```python
from build123d import *

# Parameters (mm, degrees)
CUT_EXTRUDE1_DEPTH = 2.5


with BuildPart() as part:
    # Sketch1 → Revolve1 (revolve)
    with BuildSketch(Plane(origin=(0, 0, 0), x_dir=(0, 0, -1), z_dir=(1, 0, 0))):
        with BuildLine():
            Line((-1.460769515, 0), (-2.5, 1.8))
            Line((-2.5, 1.8), (-2.5, 4.55))
            ThreePointArc((-2.5, 4.55), (-2.441421356, 4.691421356), (-2.3, 4.75))
            Line((-2.3, 4.75), (-0.833333333, 4.75))
            Line((-0.833333333, 4.75), (-0.833333333, 4.275))
            Line((-0.833333333, 4.275), (-0.683333333, 4.275))
            Line((-0.683333333, 4.275), (-0.683333333, 4.75))
            Line((-0.683333333, 4.75), (0, 4.75))
            Line((0, 4.75), (0, 2.8865))
            Line((0, 2.8865), (0.6135, 3.5))
            Line((0.6135, 3.5), (4.6865, 3.5))
            Line((4.6865, 3.5), (5.3, 2.8865))
            Line((5.3, 2.8865), (5.3, 0))
            Line((5.3, 0), (-1.460769515, 0))
        make_face()
    revolve(axis=Axis((0, 0, -5.3), (0, 0, 1)))

    # Sketch2 → Cut-Extrude1 (cut)
    with BuildSketch(Plane.XY.offset(2.5)):
        Polygon((-1.5, -0.866025404), (0, -1.732050808), (1.5, -0.866025404), (1.5, 0.866025404), (0, 1.732050808), (-1.5, 0.866025404), align=None)
    extrude(amount=-CUT_EXTRUDE1_DEPTH, mode=Mode.SUBTRACT)


solid = part.part
```
Input: part model. Units: mm. Frame: model coordinates. A direction names the side the tool comes from. Round coordinates to 2 decimals unless told otherwise and drop trailing zeros. Order: outer loops, then holes, each group sorted by start corner. A loop starts at its lowest first (then second) coordinate and runs counter-clockwise, first axis right, second up. Notation, with made-up numbers: (-2.5, 61.5) - (26.5, 61.5) arc R22 cw to (26.5, 89.5) - close; hole circle Ø9 at (7.5, 22.25). An arc over 180 degrees is marked (long way). Answer in a Markdown table with one row per item.
Item 1: Mould query, pull axis Y, two halves, no side actions, for faces 1 (the flat face through (0.76, 1.293, 1.248)), 2 (the flat face through (0, 0, 0)), 3 (the flat face through (-2, 4, 0.683)), 4 (the cylindrical face through (1.341, 3.233, -2.679)). Classes: released by +Y, released by -Y, zero draft, split by the parting line, or undercut.
Model answer:
| item | result |
|---|---|
| face 1 | undercut |
| face 2 | undercut |
| face 3 | zero draft |
| face 4 | split by the parting line |
Item 2: Pin query (flat end, axial travel): pin 1 (1 mm diameter, centred on y = 0, z = -1, fed in from -X); pin 2 (0.9 mm diameter, centred on x = 0.5, y = 0.5, fed in from +Z); pin 3 (3 mm diameter, centred on x = -2.5, z = -3, fed in from -Y). Return the tip coordinate at first contact, or that it passes through.
Model answer:
| item | result |
|---|---|
| pin 1 | stops at x = -3.5 |
| pin 2 | stops at z = 0 |
| pin 3 | stops at y = -3.35 |
Item 3: Line query: line 1 (X direction, y = 0, z = 2); line 2 (Z direction, x = 3.25, y = 2.25); line 3 (Z direction, x = -1, y = -1). Output: solid intervals per line, ascending.
Model answer:
| item | result |
|---|---|
| line 1 | x = -4.75 to -1.5, 1.5 to 4.75 |
| line 2 | z = 0 to 2.5 |
| line 3 | z = -5.3 to 0 |
Item 4: Reachability of faces 5 (the flat face through (3.1, -0.1, 0)), 6 (the flat face through (1.5, 0, 1)), 7 (the flat face through (2, 0, 2.5)) from +Z, -Z, +X, -X, +Y, -Y: full face, straight path, thin tool, end or side. Return the list, or none.
Model answer:
| item | result |
|---|---|
| face 5 | none |
| face 6 | +Z |
| face 7 | +Z, +X, -X, +Y, -Y |
Item 5: Section query A-A (z = 1.75). Return the cut outline in (x, y).
Model answer:
| item | result |
|---|---|
| outline | circle Ø9.5 at (0, 0); hole (-1.5, -0.87) - (0, -1.73) - (1.5, -0.87) - (1.5, 0.87) - (0, 1.73) - (-1.5, 0.87) - close |
Item 6: Section query C-C (z = -2.75). Return the cut outline in (x, y).
Model answer:
| item | result |
|---|---|
| outline | circle Ø7 at (0, 0) |
